from build123d import *

# Parameters (mm, degrees)
SKETCH1_W           = 116
SKETCH1_H           = 12.3
BOSS_EXTRUDE1_DEPTH = 5
SKETCH2_W           = 5
SKETCH2_H           = 5
BOSS_EXTRUDE2_DEPTH = 5
SKETCH3_W           = 72
SKETCH3_H           = 5
CUT_EXTRUDE1_DEPTH  = 17
SKETCH4_W           = 5
SKETCH4_H           = 5
BOSS_EXTRUDE3_DEPTH = 5


with BuildPart() as part:
    # Sketch1 → Boss-Extrude1 (new body)
    with BuildSketch(Plane.XY):
        Rectangle(SKETCH1_W, SKETCH1_H)
    extrude(amount=BOSS_EXTRUDE1_DEPTH)

    # Sketch2 → Boss-Extrude2 (add)
    with BuildSketch(Plane.XZ.offset(6.15)):
        with Locations((-50, 2.5)):
            Rectangle(SKETCH2_W, SKETCH2_H)
        with Locations((50, 2.5)):
            Rectangle(SKETCH2_W, SKETCH2_H)
    extrude(amount=BOSS_EXTRUDE2_DEPTH)

    # Mirror1: part across plane


with BuildPart() as part_1:
    add(part.part)
    add(part.part.mirror(Plane(origin=(-58, 6.15, 5), x_dir=(0, 0, 1), z_dir=(0, -1, 0))))

    # Sketch3 → Cut-Extrude1 (cut)
    with BuildSketch(Plane(origin=(0, 18.45, 0), x_dir=(1, 0, 0), z_dir=(0, 1, 0))):
        with Locations((0, -2.5)):
            Rectangle(SKETCH3_W, SKETCH3_H)
    extrude(amount=-CUT_EXTRUDE1_DEPTH, mode=Mode.SUBTRACT)

    # Sketch4 → Boss-Extrude3 (add)
    with BuildSketch(Plane.XZ.offset(6.15)):
        with Locations((0, 2.5)):
            Rectangle(SKETCH4_W, SKETCH4_H)
    extrude(amount=BOSS_EXTRUDE3_DEPTH)


solid = part_1.part
Verification items for the finished model (mm, model axes). A direction names the side the tool comes from. Give positions to 0.01 mm unless a question says otherwise; leave off trailing zeros. Order: outer loops, then holes, each group sorted by start corner. A loop starts at its lowest first (then second) coordinate and runs counter-clockwise, first axis right, second up. Notation, with made-up numbers: (50, -31) -> (105, -31) arc R32 cw to (105, -2) -> close; hole circle Ø9 at (81.5, 15). An arc over 180 degrees is marked (long way). Answer as CSV lines item,"result".
Q1. Sectioned sample at C-C on z = 1.75. Record the cut outline in (x, y).
Solutions:
outline,"(-58, -6.15) -> (-52.5, -6.15) -> (-52.5, -11.15) -> (-47.5, -11.15) -> (-47.5, -6.15) -> (-2.5, -6.15) -> (-2.5, -11.15) -> (2.5, -11.15) -> (2.5, -6.15) -> (47.5, -6.15) -> (47.5, -11.15) -> (52.5, -11.15) -> (52.5, -6.15) -> (58, -6.15) -> (58, 18.45) -> (52.5, 18.45) -> (52.5, 23.45) -> (47.5, 23.45) -> (47.5, 18.45) -> (36, 18.45) -> (36, 1.45) -> (-36, 1.45) -> (-36, 18.45) -> (-47.5, 18.45) -> (-47.5, 23.45) -> (-52.5, 23.45) -> (-52.5, 18.45) -> (-58, 18.45) -> close"
Q2. Sectioned sample at B-B on y = -7.5. Record the cut outline in (x, z), plus the area to 3 significant figures.
Solutions:
outline,"(-52.5, 0) -> (-47.5, 0) -> (-47.5, 5) -> (-52.5, 5) -> close; (-2.5, 0) -> (2.5, 0) -> (2.5, 5) -> (-2.5, 5) -> close; (47.5, 0) -> (52.5, 0) -> (52.5, 5) -> (47.5, 5) -> close"
area,"75.0 mm²"
Q3. Sectioned sample at D-D on x = -13. Record the cut outline in (y, z).
Solutions:
outline,"(-6.15, 0) -> (1.45, 0) -> (1.45, 5) -> (-6.15, 5) -> close"
Q4. Depth check by flat-ended pin: pin 1 (3 mm diameter, centred on x = -17, z = 1.5, fed in from -Y); pin 2 (2.5 mm diameter, centred on y = -9.5, z = 2.5, fed in from -X); pin 3 (1.5 mm diameter, centred on y = 20.5, z = 3, fed in from +X). Enter the tip coordinate at first touch or a pass-through.
Solutions:
pin 1,"stops at y = -6.15"
pin 2,"stops at x = -52.5"
pin 3,"stops at x = 52.5"
Q5. Release check for a two-part mould opening along X. For faces 1 (the flat face through (-52.5, 21, 2)), 2 (the flat face through (-50, -11.15, 3)), 3 (the flat face through (58, 6, 2)), 4 (the flat face through (47.5, 21, 2)) record: +X half, -X half, draft (parallel to the pull), parting line (faces both ways), or undercut.
Solutions:
face 1,"-X half"
face 2,"draft"
face 3,"+X half"
face 4,"undercut"
Q6. Access from +Z, -Z, +X, -X, +Y, -Y to the whole of each face (thin tool, end or side, straight path). Record for faces 5 (the flat face through (55, -6.15, 2)), 6 (the flat face through (2.5, -9, 2)), 7 (the flat face through (-47.5, 21, 2)), 8 (the flat face through (-52.5, -9, 2)).
Solutions:
face 5,"+Z, -Z, +X, -Y"
face 6,"+Z, -Z, -Y"
face 7,"+Z, -Z, +Y"
face 8,"+Z, -Z, -X, -Y"
Q7. Scan lines: probe 1 along X at (y, z) = (11, 0.3); probe 2 along X at (y, z) = (-7, 3.1); probe 3 along X at (y, z) = (21, 4.7). Record each from-to range of solid material in increasing order.
Solutions:
probe 1,"x = -58 to -36, 36 to 58"
probe 2,"x = -52.5 to -47.5, -2.5 to 2.5, 47.5 to 52.5"
probe 3,"x = -52.5 to -47.5, 47.5 to 52.5"
Q8. Sectioned sample at A-A on y = 3. Record the cut outline in (x, z).
Solutions:
outline,"(-58, 0) -> (-36, 0) -> (-36, 5) -> (-58, 5) -> close; (36, 0) -> (58, 0) -> (58, 5) -> (36, 5) -> close"
